Read the model definition and answer for the solid it produces. Units are mm, in the model's axes. A direction names the side the tool comes from. Give positions to 0.01 mm unless a question says otherwise; leave off trailing zeros. Loops run counter-clockwise (first coordinate to the right, second up) from the corner with the lowest first, then second, coordinate; pieces in that order, holes last. Notation, with made-up numbers: (64, 0) - (83, 0) arc R13 ccw to (83, 17) - close; hole circle Ø4 at (64, 13.5). An arc over 180 degrees is marked (long way). Write each question's results on one line, items separated by ' | '. Start each with the question number.
Q1. For faces 1 (the cylindrical face through (-10.25, -19.93, 18.95)), 2 (the flat face through (0, -18, -13)), 3 (the cylindrical face through (-10.063, 3.169, 20.549)), 4 (the flat face through (9, 4, -17)), determine the directions among +Z, -Z, +X, -X, +Y, -Y from which every point of the face is accessible in a straight line to the end or side of a thin tool.
Q2. The part is cut by section B-B, the plane z = 1.5. Write down the section's boundary in (x, y), plus the area to 3 significant figures.
Q3. The part is cut by section D-D, the plane z = -12. Write down the section's boundary in (x, y).
Q4. Given pin 1 (11.5 mm diameter, centred on x = 0, y = 0, fed in from +Z); pin 2 (2 mm diameter, centred on x = -9, z = -19, fed in from +Y); pin 3 (3 mm diameter, centred on x = 9, z = 19, fed in from +Y); pin 4 (8 mm diameter, centred on x = 1, z = 1, fed in from +Y), each flat-ended and moving along its own axis, determine where each tip first touches the part or whether it passes through.
Q5. Determine the mould class of faces 5 (the flat face through (9, 4, 17)), 6 (the flat face through (0, -20, 0)), 7 (the flat face through (-15, -21, 0)) for opening direction X: +X half, -X half, draft (parallel to the pull), parting line (faces both ways), or undercut.
Q6. The part is cut by section C-C, the plane x = 12.5. Write down the section's boundary in (y, z), plus the area to 3 significant figures.
Q7. Find the intervals of material crossed by line 1 (X direction, y = -21, z = 19); line 2 (Z direction, x = 8, y = 10.5); line 3 (Y direction, x = 0, z = 22), in increasing order. Write a range as from..to.
Q8. The part is cut by section A-A, the plane x = 0. Write down the section's boundary in (y, z), plus the area to 3 significant figures.
```python
from build123d import *

# Parameters (mm, degrees)
SKETCH_1_R               = 9.5
EXTRUDE_1_DEPTH          = 24
CUT_EXTRUDE_1_DEPTH      = 38.762415177
CUT_EXTRUDE_1_DEPTH_BACK = 38.762415177
SKETCH_2_W               = 30
SKETCH_2_H               = 69.949963181
SKETCH_4_R               = 10.55
CUT_EXTRUDE_3_DEPTH      = 7
CHAMFER_2_SIZE           = 4
HOLE_WIZARD_M3_1_D       = 2.5
HOLE_WIZARD_M3_1_DEPTH   = 10
HOLE_WIZARD_M3_1_TIP     = 0.751075774


with BuildPart() as part:
    # 草图1 → 凸台-拉伸1 (new, symmetric)
    with BuildSketch(Plane.XY):
        with BuildLine():
            Line((-15, -25), (-15, 0))
            ThreePointArc((-15, 0), (0, 15), (15, 0))
            Line((15, 0), (15, -25))
            Line((15, -25), (-15, -25))
        make_face()
        Circle(SKETCH_1_R, mode=Mode.SUBTRACT)
    extrude(amount=EXTRUDE_1_DEPTH, both=True)

    # 草图2 → 切除-拉伸1 (cut, two sides: drawn at the far end of the back side and taken through both)
    with BuildSketch(Plane(origin=(0, 0, 0), x_dir=(0, 0, -1), z_dir=(1, 0, 0)).offset(-CUT_EXTRUDE_1_DEPTH_BACK)):
        with Locations((0, 14.974981591)):
            Rectangle(SKETCH_2_W, SKETCH_2_H)
    extrude(amount=CUT_EXTRUDE_1_DEPTH + CUT_EXTRUDE_1_DEPTH_BACK, mode=Mode.SUBTRACT)

    # 草图4 → 切除-拉伸3 (cut)
    with BuildSketch(Plane(origin=(0, 0, -24), x_dir=(-1, 0, 0), z_dir=(0, 0, -1))):
        Circle(SKETCH_4_R)
    cut_extrude_3 = extrude(amount=-CUT_EXTRUDE_3_DEPTH, mode=Mode.SUBTRACT)

    # 倒角2
    chamfer_2_edges = [part.edges().sort_by_distance(p)[0] for p in [
        (0, -20, 15),
        (0, -20, -15),
    ]]
    chamfer(chamfer_2_edges, length=CHAMFER_2_SIZE)

    # M3 螺纹孔1
    with Locations(Plane(origin=(0, -25, 0), x_dir=(-1, 0, 0), z_dir=(0, -1, 0))):
        with Locations((9, -19), (-9, -19), (9, 19), (-9, 19)):
            Hole(HOLE_WIZARD_M3_1_D / 2, depth=HOLE_WIZARD_M3_1_DEPTH)
            with Locations((0, 0, -(HOLE_WIZARD_M3_1_DEPTH + HOLE_WIZARD_M3_1_TIP / 2))):  # 118° drill point
                Cone(0, HOLE_WIZARD_M3_1_D / 2, HOLE_WIZARD_M3_1_TIP, mode=Mode.SUBTRACT)

    # 镜向1: 切除-拉伸3 across plane
    add(cut_extrude_3.mirror(Plane.XY), mode=Mode.SUBTRACT)


solid = part.part
```
Check sheet entries:
1) face 1: -Y | face 2: +X, -X, +Y | face 3: +Z | face 4: -Z
2) outline: (-15, -25) - (15, -25) - (15, -20) - (-15, -20) - close | area: 150 mm^2
3) outline: (-15, -25) - (15, -25) - (15, -19) - (-15, -19) - close
4) pin 1: passes through | pin 2: stops at y = 12.69 | pin 3: stops at y = 12.99 | pin 4: stops at y = -20
5) face 5: undercut | face 6: draft | face 7: -X half
6) outline: (-25, -24) - (8.29, -24) - (8.29, -15) - (-16, -15) - (-20, -11) - (-20, 11) - (-16, 15) - (8.29, 15) - (8.29, 24) - (-25, 24) - close | area: 765 mm^2
7) line 1: x = -15..-10.25, -7.75..7.75, 10.25..15 | line 2: z = -24..-15, 15..24 | line 3: y = -25..-10.55, 10.55..15
8) outline: (-25, -24) - (-10.55, -24) - (-10.55, -17) - (-9.5, -17) - (-9.5, -15) - (-16, -15) - (-20, -11) - (-20, 11) - (-16, 15) - (-9.5, 15) - (-9.5, 17) - (-10.55, 17) - (-10.55, 24) - (-25, 24) - close; (9.5, -17) - (10.55, -17) - (10.55, -24) - (15, -24) - (15, -15) - (9.5, -15) - close; (9.5, 15) - (15, 15) - (15, 24) - (10.55, 24) - (10.55, 17) - (9.5, 17) - close | area: 515 mm^2
